from build123d import *

# Parameters (mm, degrees)
SKETCH1_R           = 8
SKETCH1_R_2         = 4
BOSS_EXTRUDE1_DEPTH = 8
SKETCH2_R           = 16
SKETCH2_R_2         = 1.95
BOSS_EXTRUDE2_DEPTH = 2
SKETCH3_R           = 2
CUT_EXTRUDE1_DEPTH  = 10


with BuildPart() as part:
    # Sketch1 → Boss-Extrude1 (new body)
    with BuildSketch(Plane.XY):
        Circle(SKETCH1_R)
        Circle(SKETCH1_R_2, mode=Mode.SUBTRACT)
    extrude(amount=BOSS_EXTRUDE1_DEPTH)

    # Sketch2 → Boss-Extrude2 (add)
    with BuildSketch(Plane.XY):
        Circle(SKETCH2_R)
        with Locations((12, 0)):
            Circle(SKETCH2_R_2, mode=Mode.SUBTRACT)
        with Locations((0, -12)):
            Circle(SKETCH2_R_2, mode=Mode.SUBTRACT)
        with Locations((-12, 0)):
            Circle(SKETCH2_R_2, mode=Mode.SUBTRACT)
        with Locations((0, 12)):
            Circle(SKETCH2_R_2, mode=Mode.SUBTRACT)
    extrude(amount=BOSS_EXTRUDE2_DEPTH)

    # Sketch3 → Cut-Extrude1 (cut, symmetric)
    with BuildSketch(Plane(origin=(0, 0, 0), x_dir=(1, 0, 0), z_dir=(0, 1, 0))):
        with Locations(Location((0, -5, 0), (0, 0, 270))):
            Circle(SKETCH3_R)
    extrude(amount=CUT_EXTRUDE1_DEPTH, both=True, mode=Mode.SUBTRACT)


solid = part.part
Check sheet for the modelled part. Datum: model origin and axes. Units: mm. A direction names the side the tool comes from. Round coordinates to 2 decimals unless told otherwise and drop trailing zeros. Order: outer loops, then holes, each group sorted by start corner. A loop starts at its lowest first (then second) coordinate and runs counter-clockwise, first axis right, second up.
(1) Access from +Z, -Z, +X, -X, +Y, -Y to the whole of each face (thin tool, end or side, straight path). Record for faces 1 (the cylindrical face through (-1.547, 10.813, 0.986)), 2 (the cylindrical face through (3.69, -7.1, 4.96)).
(2) Cross-section at D-D, the plane y = -10.5. Enter the section's corners in (x, z), and give its area (3 significant figures).
(3) Cross-section at A-A, the plane x = 0. Enter the section's corners in (y, z), and give its area (3 significant figures).
(4) Scan lines: probe 1 along Y at (x, z) = (0, 1.45); probe 2 along Z at (x, y) = (-10, 2); probe 3 along X at (y, z) = (0, 3). Record each from-to range of solid material in increasing order.
(5) Cross-section at B-B, the plane z = 6.25. Enter the section's corners in (x, y).
(6) Draft check along X on faces 3 (the cylindrical face through (-3.47, -15.62, 0.99)), 4 (the cylindrical face through (-0.766, 5.767, 6.847)), 5 (the flat face through (-3.8, 7.3, 2)). Enter one of: pulls with the +X half, pulls with the -X half, needs draft (parallel to the pull), parting line crosses it, or undercut.
(7) Go/stop test with flat-tipped pins: P1, Ø3, axis at x = 12, y = 0, coming from the +Z side; P2, Ø4, axis at x = -0.5, y = 0.5, coming from the +Z side; P3, Ø4.5, axis at x = 0, z = 5, coming from the -Y side; P4, Ø1.5, axis at x = 10.5, z = 2, coming from the -Y side. Record where each tip stops, or that it passes through.
(8) Cross-section at C-C, the plane y = 0. Enter the section's corners in (x, z).
Check sheet entries:
1. face 1: +Z, -Z
1. face 2: +Z
2. outline: (-12.07, 0) - (-1.25, 0) - (-1.25, 2) - (-12.07, 2) - close; (1.25, 0) - (12.07, 0) - (12.07, 2) - (1.25, 2) - close
2. area: 43.3 mm2
3. outline: (-16, 0) - (-13.95, 0) - (-13.95, 2) - (-16, 2) - close; (-10.05, 0) - (10.05, 0) - (10.05, 2) - (8, 2) - (8, 3) - (4, 3) - (4, 2) - (-4, 2) - (-4, 3) - (-8, 3) - (-8, 2) - (-10.05, 2) - close; (-8, 7) - (-4, 7) - (-4, 8) - (-8, 8) - close; (4, 7) - (8, 7) - (8, 8) - (4, 8) - close; (13.95, 0) - (16, 0) - (16, 2) - (13.95, 2) - close
3. area: 64.4 mm2
4. probe 1: y = -16 to -13.95, -10.05 to 10.05, 13.95 to 16
4. probe 2: z = 0 to 2
4. probe 3: x = -8 to -4, 4 to 8
5. outline: (-1.56, -7.85) - (-1.56, -3.68) arc R4 cw to (-1.56, 3.68) - (-1.56, 7.85) arc R8 ccw to start; (1.56, -7.85) arc R8 ccw to (1.56, 7.85) - (1.56, 3.68) arc R4 cw to (1.56, -3.68) - close
6. face 3: parting line crosses it
6. face 4: undercut
6. face 5: needs draft
7. P1: passes through
7. P2: stops at z = 2
7. P3: stops at y = -8
7. P4: stops at y = -12.69
8. outline: (-16, 0) - (-13.95, 0) - (-13.95, 2) - (-16, 2) - close; (-10.05, 0) - (10.05, 0) - (10.05, 2) - (8, 2) - (8, 8) - (4, 8) - (4, 2) - (-4, 2) - (-4, 8) - (-8, 8) - (-8, 2) - (-10.05, 2) - close; (13.95, 0) - (16, 0) - (16, 2) - (13.95, 2) - close
